Input: part model. Units: mm. Frame: model coordinates. Give positions to 0.01 mm unless a question says otherwise; leave off trailing zeros. Loops run counter-clockwise (first coordinate to the right, second up) from the corner with the lowest first, then second, coordinate; pieces in that order, holes last. Notation, with made-up numbers: (50, 21) - (109, 21) arc R10 cw to (109, 27) - close; hole circle Ø7 at (82.5, 0). An arc over 180 degrees is marked (long way). Answer as a JSON object with one key per item and string values. Group by question number.
(1) Section query D-D (y = 5). Count the separate pieces of the cut face and the enclosed holes in it, plus the area to 3 significant figures.
(2) Section query C-C (z = -60). Return loops of the section in (x, y).
(3) Pin query (flat end, axial travel): P1, Ø5, axis at x = -20, z = -60, coming from the -Y side; P2, Ø8, axis at x = -60, z = -20, coming from the +Y side. Return the tip coordinate at first contact, or that it passes through.
(4) Section query A-A (x = -20). Return loops of the section in (y, z), plus the area to 3 significant figures.
(5) Material intervals for L1, parallel to Z at x = -60, y = 1.75; L2, parallel to X at y = 5.5, z = -74; L3, parallel to Z at x = -58, y = 5.75, sorted ascending.
(6) Section query B-B (z = -40). Return loops of the section in (x, y) (3 decimals).
Autodesk Inventor part; units mm, degrees
ref_plane "YZ Plane" through (0, 0, 0) normal (1, 0, 0) x (0, 1, 0)
ref_plane "XZ Plane" through (0, 0, 0) normal (0, 1, 0) x (-1, 0, 0)
ref_plane "XY Plane" through (0, 0, 0) normal (0, 0, 1) x (1, 0, 0)
sketch "Sketch1" plane through (0, 0, 0) normal (0, 1, 0) x (-1, 0, 0)
  circle A0 centre (20, -20) radius 18.1118 construction
  line L0 (0, 0) -> (80, 0)
  line L1 (80, 0) -> (80, -80)
  line L2 (80, -80) -> (0, -80)
  line L3 (0, -80) -> (0, 0)
  line L4 (40, 0) -> (40, -40) construction
  line L5 (40, -40) -> (80, -40) construction
  line L6 (40, -40) -> (40, -80) construction
  line L7 (40, -40) -> (0, -40) construction
  circle A1 centre (40, -40) radius 1.715
  line L8 (40, -40) -> (0, 0) construction
  circle A2 centre (4.6447, -4.6447) radius 1.715
  circle A3 centre (75.3553, -4.6447) radius 1.715
  circle A4 centre (4.6447, -75.3553) radius 1.715
  circle A5 centre (75.3553, -75.3553) radius 1.715
  circle A6 centre (20, -20) radius 3.15
  circle A7 centre (60, -20) radius 3.15
  circle A8 centre (20, -60) radius 3.15
  circle A9 centre (60, -60) radius 3.15
  point P0 (40, -20)
  point P1 (20, -40)
  dimension "d0" = 36.2235
  dimension "d1" = 80
  dimension "d2" = 80
  dimension "d13" = 3.43
  dimension "d14" = 3.43
  dimension "d15" = 50
  dimension "d16" = 6.3
extrude "Extrusion3" add sketch "Sketch1" along normal blind 6.39
equation "\"d0\" = SiliconeRingDiameter"
equation "\"d1\" = VccumCoverSize"
equation "\"d2\" = VccumCoverSize"
equation "\"d13\" = HoldScrewDiameter"
equation "\"d14\" = HoldScrewDiameter"
equation "\"d16\" = DowlDiameter"
equation "\"d17\" = WoodThickness"
equation "\"BearingHolderHeight\" = 13.1"
equation "\"SiliconeRingDiameter\" = 0.75 * CouplingDiameter + 1.5 * BearingHolderHeight"
equation "\"DowlDiameter\" = 6.3"
equation "\"HoldScrewDiameter\" = 3.43"
equation "\"VccumCoverSize\" = 80"
properties part number "MotorSiliconeMold_1" material "MDF Medium Density Fiberboard"
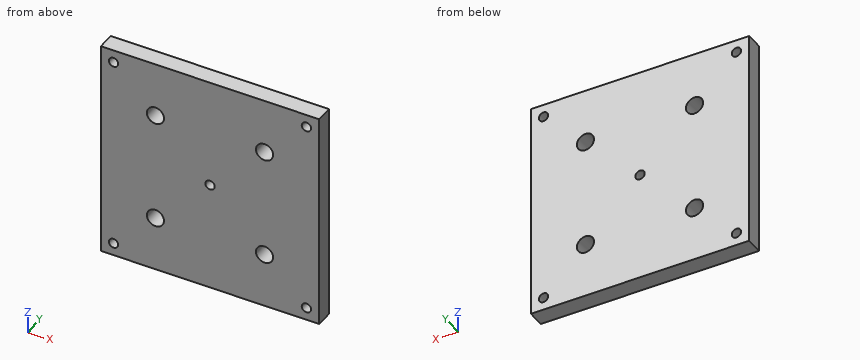
Recorded:
{
 "1": {"separate pieces": "1", "enclosed holes": "9", "area": "6,230 mm^2"},
 "2": {"outline": "(-80, 0) - (-63.15, 0) - (-63.15, 6.39) - (-80, 6.39) - close; (-56.85, 0) - (-23.15, 0) - (-23.15, 6.39) - (-56.85, 6.39) - close; (-16.85, 0) - (0, 0) - (0, 6.39) - (-16.85, 6.39) - close"},
 "3": {"P1": "passes through", "P2": "stops at y = 6.39"},
 "4": {"outline": "(0, -80) - (6.39, -80) - (6.39, -63.15) - (0, -63.15) - close; (0, -56.85) - (6.39, -56.85) - (6.39, -23.15) - (0, -23.15) - close; (0, -16.85) - (6.39, -16.85) - (6.39, 0) - (0, 0) - close", "area": "431 mm^2"},
 "5": {"L1": "z = -80 to -63.15, -56.85 to -23.15, -16.85 to 0", "L2": "x = -80 to -76.41, -74.3 to -5.7, -3.59 to 0", "L3": "z = -80 to -62.43, -57.57 to -22.43, -17.57 to 0"},
 "6": {"outline": "(-80, 0) - (-41.715, 0) - (-41.715, 6.39) - (-80, 6.39) - close; (-38.285, 0) - (0, 0) - (0, 6.39) - (-38.285, 6.39) - close"}
}
